Job drawing, mm, ordinate dimensions from the low corner. One solid piece. A direction names the side the tool comes from. Round coordinates to 2 decimals unless told otherwise and drop trailing zeros. Write each loop counter-clockwise with the first axis right and the second up, starting at its lowest first coordinate (ties: lowest second). Pieces come first, ordered by that corner, then holes.
1) Saw through at A-A on z = 36.5. Write the cut outline in (x, y), and give its area (3 significant figures).
2) Which spindle directions (+Z, -Z, +X, -X, +Y, -Y) get a long thin tool onto all of the face, cutting with end or side? Do the marked faces 1 and 2. Say none if no direction does.
3) Saw through at B-B on y = 100. Write the cut outline in (x, z).
4) Saw through at C-C on x = 100. Count the separate pieces of the cut face and the enclosed holes in it, and give its area (3 significant figures).
5) Flat gauge pins, fed straight in: pin 1 (2.5 mm diameter, centred on y = 117.5, z = 52, fed in from -X); pin 2 (8.5 mm diameter, centred on x = 100, z = 60, fed in from +Y); pin 3 (2.5 mm diameter, centred on y = 84, z = 67.5, fed in from +X); pin 4 (15 mm diameter, centred on x = 102.5, z = 72, fed in from -Y). Where does each tip first touch, or does it go through?
6) Drill centre lines: L1, parallel to X at y = 114.5, z = 60; L2, parallel to Z at x = 100, y = 115; L3, parallel to Z at x = 97, y = 179. Where is each one in solid material? Low to high.
7) Saw through at D-D on z = 60. Write the cut outline in (x, y), and give its area (3 significant figures).
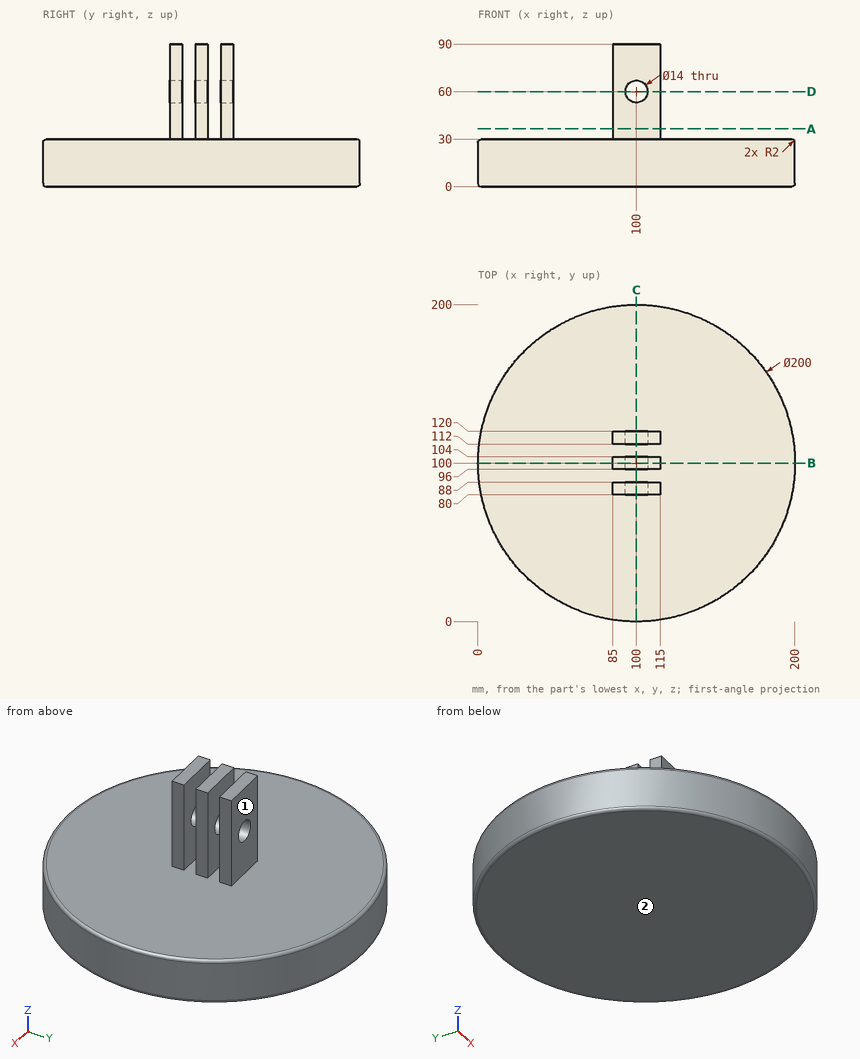
Completed:
1. outline: (85, 80) - (115, 80) - (115, 88) - (85, 88) - close; (85, 96) - (115, 96) - (115, 104) - (85, 104) - close; (85, 112) - (115, 112) - (115, 120) - (85, 120) - close
1. area: 720 mm2
2. face 1: +Z, +X, -X, +Y
2. face 2: -Z, +X, -X, +Y, -Y
3. outline: (0, 2) arc R2 ccw to (2, 0) - (198, 0) arc R2 ccw to (200, 2) - (200, 28) arc R2 ccw to (198, 30) - (115, 30) - (115, 90) - (85, 90) - (85, 30) - (2, 30) arc R2 ccw to (0, 28) - close; hole circle Ø14 at (100, 60)
4. separate pieces: 4
4. enclosed holes: 0
4. area: 7,100 mm2
5. pin 1: stops at x = 85
5. pin 2: passes through
5. pin 3: stops at x = 115
5. pin 4: stops at y = 80
6. L1: x = 85 to 93, 107 to 115
6. L2: z = 0 to 53, 67 to 90
6. L3: z = 0 to 30
7. outline: (85, 80) - (93, 80) - (93, 88) - (85, 88) - close; (85, 96) - (93, 96) - (93, 104) - (85, 104) - close; (85, 112) - (93, 112) - (93, 120) - (85, 120) - close; (107, 80) - (115, 80) - (115, 88) - (107, 88) - close; (107, 96) - (115, 96) - (115, 104) - (107, 104) - close; (107, 112) - (115, 112) - (115, 120) - (107, 120) - close
7. area: 384 mm2
